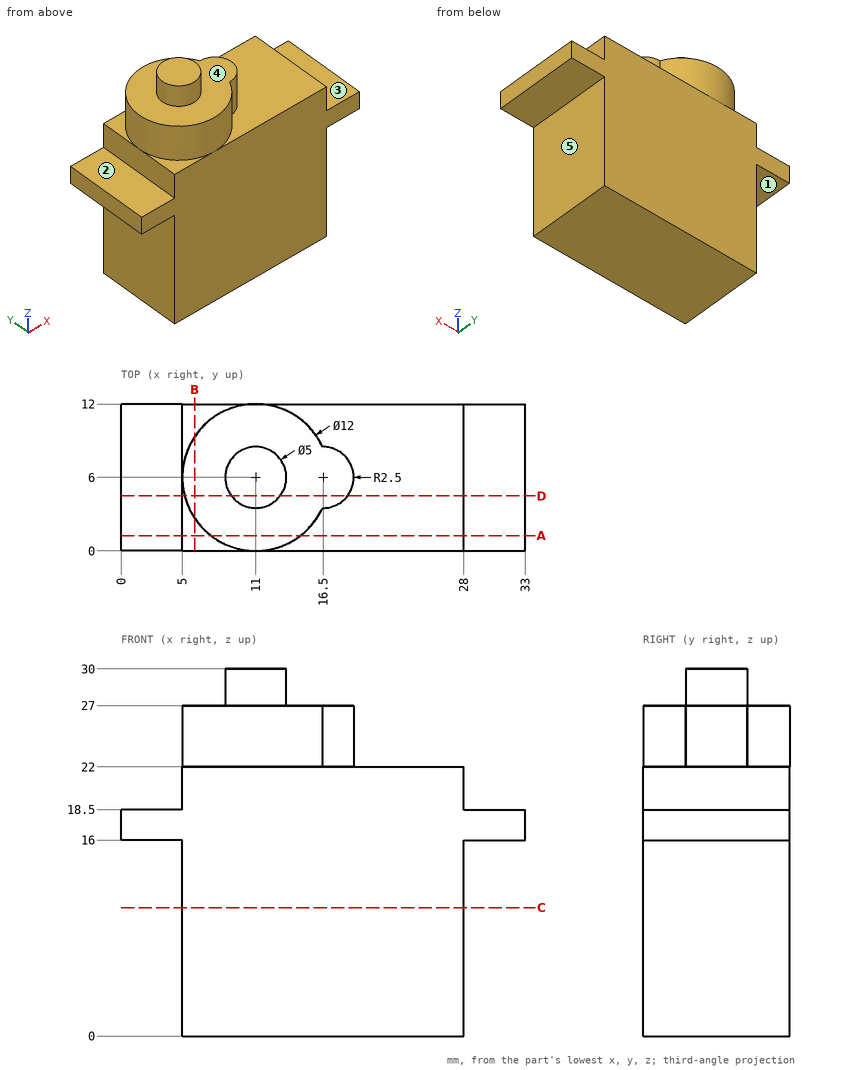
Print and shaded views of the part. All mm, measured from the part's lowest x, y and z. A direction names the side the tool comes from. Round coordinates to 2 decimals unless told otherwise and drop trailing zeros. Order: outer loops, then holes, each group sorted by start corner. A loop starts at its lowest first (then second) coordinate and runs counter-clockwise, first axis right, second up. Notation, with made-up numbers: (-7.75, 54.5) - (7.25, 54.5) arc R24 cw to (7.25, 85.5) - close; hole circle Ø1 at (-37.75, 13.5). An arc over 180 degrees is marked (long way). Use a Markdown table: item, result.
1) Wall check: L1, parallel to X at y = 6, z = 19.75; L2, parallel to Z at x = 31, y = 4.5; L3, parallel to Z at x = 23.5, y = 2.5. Give the ranges that are in metal, low to high.
Recorded:
| item | result |
|---|---|
| L1 | x = 5 to 28 |
| L2 | z = 16 to 18.5 |
| L3 | z = 0 to 22 |
2) Saw through at A-A on y = 1.25. Write the cut outline in (x, z).
Recorded:
| item | result |
|---|---|
| outline | (0, 16) - (5, 16) - (5, 0) - (28, 0) - (28, 16) - (33, 16) - (33, 18.5) - (28, 18.5) - (28, 22) - (14.67, 22) - (14.67, 27) - (7.33, 27) - (7.33, 22) - (5, 22) - (5, 18.5) - (0, 18.5) - close |
3) Saw through at C-C on z = 10.5. Write the cut outline in (x, y).
Recorded:
| item | result |
|---|---|
| outline | (5, 0) - (28, 0) - (28, 12) - (5, 12) - close |
4) Tool access for the marked faces 1, 2, 3, 4 and 5: list every direction of +Z, -Z, +X, -X, +Y, -Y with a clear straight run to the whole face (end or side of a thin tool).
Recorded:
| item | result |
|---|---|
| face 1 | -Z, -X, +Y, -Y |
| face 2 | +Z, -X, +Y, -Y |
| face 3 | +Z, +X, +Y, -Y |
| face 4 | +Z |
| face 5 | -Z, +X, +Y, -Y |
5) Flat gauge pins, fed straight in: pin 1 Ø1.5 at (x, y) = (27.5, 1.5) entering from +Z; pin 2 Ø3 at (x, y) = (7.5, 3) entering from +Z; pin 3 Ø3.5 at (y, z) = (5.5, 6) entering from +X. Where does each tip first touch, or does it go through?
Recorded:
| item | result |
|---|---|
| pin 1 | stops at z = 22 |
| pin 2 | stops at z = 27 |
| pin 3 | stops at x = 28 |
6) Saw through at D-D on y = 4.5. Write the cut outline in (x, z).
Recorded:
| item | result |
|---|---|
| outline | (0, 16) - (5, 16) - (5, 0) - (28, 0) - (28, 16) - (33, 16) - (33, 18.5) - (28, 18.5) - (28, 22) - (18.5, 22) - (18.5, 27) - (13, 27) - (13, 30) - (9, 30) - (9, 27) - (5.19, 27) - (5.19, 22) - (5, 22) - (5, 18.5) - (0, 18.5) - close |
7) Saw through at B-B on x = 6. Write the cut outline in (y, z), and give its area (3 significant figures).
Recorded:
| item | result |
|---|---|
| outline | (0, 0) - (12, 0) - (12, 22) - (9.32, 22) - (9.32, 27) - (2.68, 27) - (2.68, 22) - (0, 22) - close |
| area | 297 mm² |
